from build123d import *

# Parameters (mm, degrees)
CUT_EXTRUDE3_DEPTH      = 20
CUT_EXTRUDE3_DEPTH_BACK = 200.5


with BuildPart() as part:
    # Sketch1 → Revolve1 (revolve)
    with BuildSketch(Plane.XY):
        with BuildLine():
            Line((4, 0), (-4, 0))
            Line((-4, 0), (-8.408174518, 25))
            Line((-8.408174518, 25), (-11.872276133, 31))
            ThreePointArc((-11.872276133, 31), (0, 35.931604452), (11.872276133, 31))
            Line((11.872276133, 31), (8.408174518, 25))
            Line((8.408174518, 25), (4, 0))
        make_face()
    revolve(axis=Axis((-4, -5, 0), (1, 0, 0)))

    # Sketch2 → Cut-Extrude3 (cut, two sides)
    with BuildSketch(Plane(origin=(0, 0, 0), x_dir=(0, 0, -1), z_dir=(1, 0, 0))) as cut_extrude3_sk:
        with BuildLine():
            Line((-1, -5), (1, -5))
            Line((1, -5), (1, 2.937253933))
            ThreePointArc((1, 2.937253933), (0, 3), (-1, 2.937253933))
            Line((-1, 2.937253933), (-1, -5))
        make_face()
    extrude(amount=CUT_EXTRUDE3_DEPTH, mode=Mode.SUBTRACT)
    extrude(cut_extrude3_sk.sketch, amount=-CUT_EXTRUDE3_DEPTH_BACK, mode=Mode.SUBTRACT)


solid = part.part
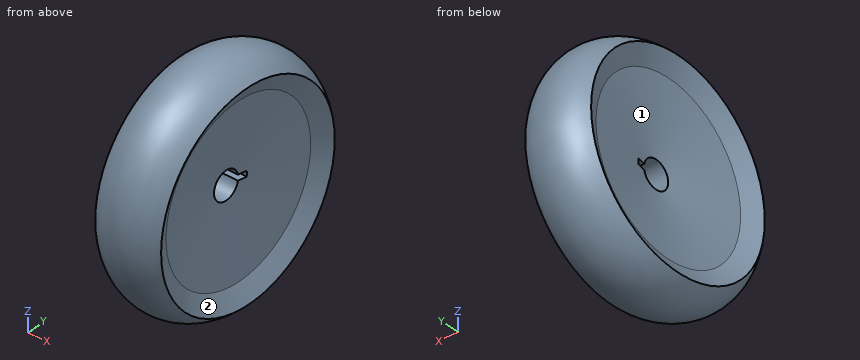
Geometry: final body of the model. Coordinates: model frame, mm. Face numbers are marked on the shaded views. Give positions to 0.01 mm unless a question says otherwise; leave off trailing zeros. Loops run counter-clockwise (first coordinate to the right, second up) from the corner with the lowest first, then second, coordinate; pieces in that order, holes last. Notation, with made-up numbers: (-33.75, 76.5) -> (-25.75, 76.5) arc R25 ccw to (-25.75, 115.5) -> close; hole circle Ø9 at (9, 39). An arc over 180 degrees is marked (long way). Put each result on its own line as item: value.
1. Pin query (flat end, axial travel): P1, Ø1, axis at x = 6.5, z = 12.5, coming from the -Y side (3 decimals); P2, Ø4, axis at y = 7.5, z = 17, coming from the +X side; P3, Ø3, axis at x = 5.5, z = 25, coming from the -Y side. Return the tip coordinate at first contact, or that it passes through.
Taken from the geometry:
P1: stops at y = -42.865
P2: stops at x = 7.19
P3: stops at y = -37.53
2. Ray query, line 1 along Z through (x, y) = (-0.5, -5); line 2 along Z through (x, y) = (8.5, -13); line 3 along Y through (x, z) = (8.75, -8). Return the intervals inside material, ascending. Write a range as [from, to].
Taken from the geometry:
line 1: z = [-40.92, -5], [5, 40.92]
line 2: z = [-37.78, -29.08], [29.08, 37.78]
line 3: y = [-42.62, -34.53], [24.53, 32.62]
3. Cut plane A-A (z = 0). Return the cut outline in (x, y).
Taken from the geometry:
outline: (-11.87, -41) arc R16.76 ccw to (11.87, -41) -> (8.41, -35) -> (4, -10) -> (-4, -10) -> (-8.41, -35) -> close; (-11.87, 31) -> (-8.41, 25) -> (-4.53, 3) -> (4.53, 3) -> (8.41, 25) -> (11.87, 31) arc R16.76 ccw to start
4. Cut plane B-B (y = -5). Return the cut outline in (x, z).
Taken from the geometry:
outline: (-11.87, -36) arc R16.76 ccw to (11.87, -36) -> (8.41, -30) -> (4, -5) -> (-4, -5) -> (-8.41, -30) -> close; (-11.87, 36) -> (-8.41, 30) -> (-4, 5) -> (4, 5) -> (8.41, 30) -> (11.87, 36) arc R16.76 ccw to start
5. Pull-direction query (Y, two-part tool) for the marked faces 1 and 2; classes: released by +Y, released by -Y, zero draft, split by the parting line, or undercut.
Taken from the geometry:
face 1: undercut
face 2: undercut
6. Cut plane C-C (x = 0). Return the cut outline in (y, z).
Taken from the geometry:
outline: circle Ø81.86 at (-5, 0); hole (-0.1, -1) -> (2.94, -1) arc R8 ccw to (2.94, 1) -> (-0.1, 1) arc R5 ccw (long way) to start
